Design review of the part shown in the three views and the two pictorial views. Dimensions are in mm from the part's minimum x, y and z. A direction names the side the tool comes from. Round coordinates to 2 decimals unless told otherwise and drop trailing zeros. Write each loop counter-clockwise with the first axis right and the second up, starting at its lowest first coordinate (ties: lowest second). Pieces come first, ordered by that corner, then holes. Notation, with made-up numbers: (87.25, -22.5) -> (124.25, -22.5) arc R31 ccw to (124.25, 16.5) -> close; hole circle Ø2 at (26, 10). An arc over 180 degrees is marked (long way). Answer as a JSON object with one key per item and string values. Group by question number.
1) Machinability: for the marked faces 1, 2, 3 and 4, which of the approach directions +Z, -Z, +X, -X, +Y, -Y give a long, thin tool a straight path to every point of the face, cutting with its end or side? Answer none if there is none.
2) To check wall thickness, follow probe 1 along X at (y, z) = (94.25, 75); probe 2 along Z at (x, y) = (180, 86.5); probe 3 along X at (y, z) = (16, 10). State the ranges of each line that lie inside material, in increasing order. Write a range as [from, to].
3) Insertion check: pin 1 Ø9.5 at (x, z) = (40, 75) entering from -Y; pin 2 Ø11 at (y, z) = (92.5, 46.5) entering from +X; pin 3 Ø12 at (x, y) = (86, 95) entering from -Z; pin 4 Ø10 at (x, z) = (194.5, 70) entering from -Y. Each pin has a flat end and moves straight along its axis. Give the tip position at first contact, or say it passes through.
4) We need section C-C, the plane x = 40. Write out the cut boundary in (y, z), then the cut area to 3 significant figures.
5) We need section B-B, the plane z = 75. Count the separate pieces of the cut face and the enclosed holes in it, then the cut area to 3 significant figures.
6) We need section D-D, the plane x = 16.5. Write out the cut boundary in (y, z).
7) We need section A-A, the plane y = 53.5. Write out the cut boundary in (x, z), then the cut area to 3 significant figures.
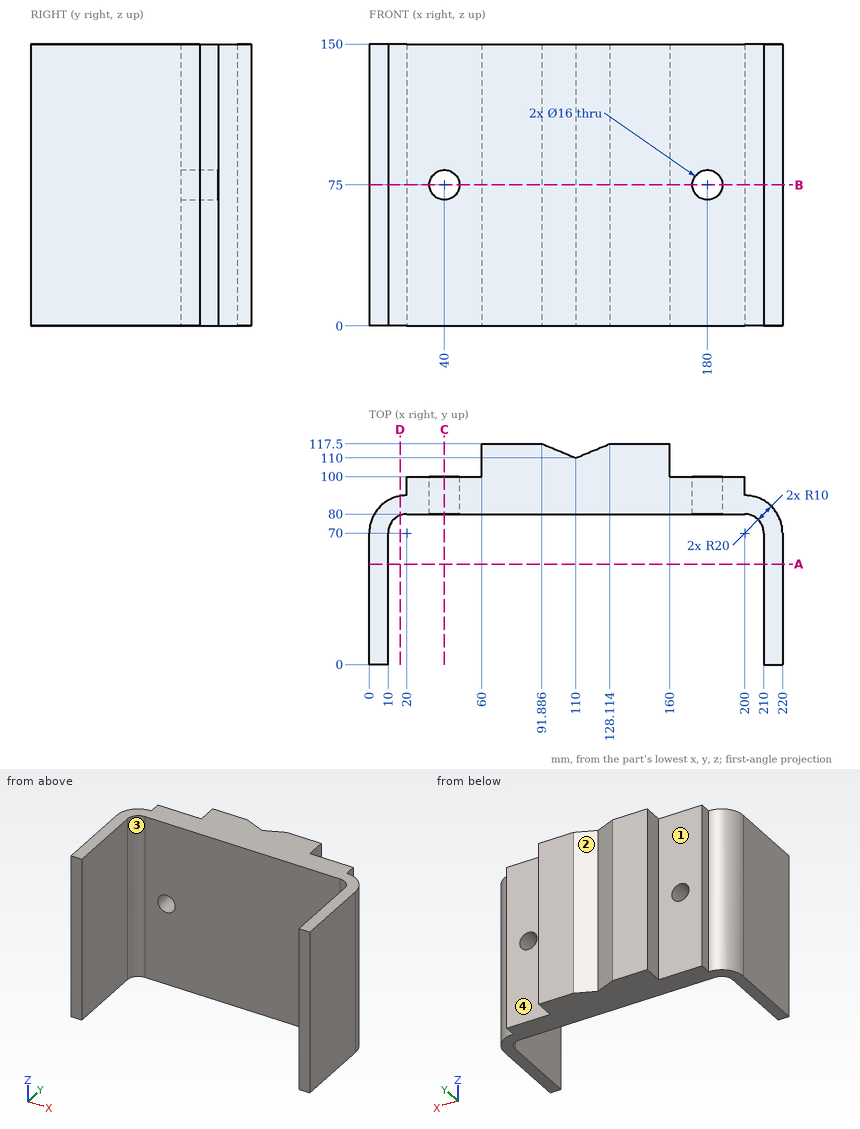
Here are the results:
{
 "1": {"face 1": "+Z, -Z, -X, +Y", "face 2": "+Z, -Z, +Y", "face 3": "+Z, -Z, -Y", "face 4": "+Z, -Z, +X, +Y"},
 "2": {"probe 1": "x = [20, 32], [48, 172], [188, 200]", "probe 2": "z = [0, 67], [83, 150]", "probe 3": "x = [0, 10], [210, 220]"},
 "3": {"pin 1": "passes through", "pin 2": "stops at x = 210.54", "pin 3": "stops at z = 0", "pin 4": "stops at y = 80"},
 "4": {"outline": "(80, 0) -> (100, 0) -> (100, 67) -> (80, 67) -> close; (80, 83) -> (100, 83) -> (100, 150) -> (80, 150) -> close", "area": "2,680 mm^2"},
 "5": {"separate pieces": "3", "enclosed holes": "0", "area": "6,450 mm^2"},
 "6": {"outline": "(79.37, 0) -> (89.69, 0) -> (89.69, 150) -> (79.37, 150) -> close"},
 "7": {"outline": "(0, 0) -> (10, 0) -> (10, 150) -> (0, 150) -> close; (210, 0) -> (220, 0) -> (220, 150) -> (210, 150) -> close", "area": "3,000 mm^2"}
}
